from build123d import *


with BuildPart() as f1:
    # F0 (on Front) → F1 (revolve)
    with BuildSketch(Plane.XZ):
        Polygon((0, 34.925), (0, 31.75), (9.525, 31.75), (12.7, 31.75), (12.7, 34.925), (8.2938163461, 34.925), align=None)
        with BuildLine():
            Line((0, 50.8), (0, 34.925))
            Line((0, 34.925), (8.2938163461, 34.925))
            add(Edge.make_bspline(
                [(8.2938163461, 34.925), (8.8119155958, 35.9296320353), (10.3377018861, 37.6445575669), (11.8497804306, 40.251445047), (11.4775968675, 43.983221376), (10.0574266195, 46.7037851398), (7.7383380098, 48.5934290358), (5.9489654676, 49.9634460717), (3.4584093672, 50.868512047), (1.1692841349, 50.6999896772), (0, 50.8)],
                knots=[0, 0, 0, 0, 0.1331073225, 0.2566905305, 0.3928132468, 0.5191817197, 0.6423867268, 0.7502366215, 0.865279277, 1, 1, 1, 1], degree=3))
        make_face()
        with BuildLine():
            Line((0, 31.75), (0, 0))
            Line((0, 0), (19.05, 0))
            Line((19.05, 0), (19.05, 12.7))
            add(Edge.make_bspline(
                [(19.05, 12.7), (15.6508699467, 13.689246051), (10.4916904552, 17.7065910039), (7.3409641587, 20.4386906172), (6.3373062495, 26.3121345815), (10.1150269054, 30.4028265886), (9.525, 31.75)],
                knots=[0, 0, 0, 0, 0.3180499089, 0.5206308145, 0.7551272901, 1, 1, 1, 1], degree=3))
            Line((9.525, 31.75), (0, 31.75))
        make_face()
    revolve(axis=Axis((0, 0, 25.4), (0, 0, 1)))


solid = f1.part
Read the model definition and answer for the solid it produces. Units are mm, in the model's axes. A direction names the side the tool comes from. Coordinates: 2 decimals unless noted, no trailing zeros. Order: outer loops, then holes, each group sorted by start corner. A loop starts at its lowest first (then second) coordinate and runs counter-clockwise, first axis right, second up. Notation, with made-up numbers: M -5,86 L 8,86 A19 cw 8,96 Z; hole C 76.5,20 d8. An arc over 180 degrees is marked long. Put each result on its own line as item: value. Start each with the question number.
Item 1: Section A-A, the plane x = -10.5 is taken. Count the separate pieces of the cut face and the enclosed holes in it, plus the area to 3 significant figures.
Item 2: The mould has two halves that part along Z. Classify faces 3 (the face through (-2.75, -12.4, 33.36)), 4 (the face through (0, 0, 0)), 5 (the face through (-5, 9, 31.75)): +Z half, -Z half, draft (parallel to the pull), parting line (faces both ways), or undercut.
Item 3: Section B-B, the plane z = 6 is taken. Determine the outline of the cut face in (x, y), plus the area to 3 significant figures.
Item 4: Section D-D, the plane z = 33 is taken. Determine the outline of the cut face in (x, y).
Item 5: Given pin 1 Ø6 at (x, z) = (5.5, 41.5) entering from -Y; pin 2 Ø10 at (x, y) = (-12.5, -13.5) entering from +Z; pin 3 Ø6 at (x, y) = (1.5, 13.5) entering from +Z, each flat-ended and moving along its own axis, determine where each tip first touches the part or whether it passes through.
Item 6: For faces 1 (the face through (-15.12, -11.59, 6.44)), 2 (the face through (3, -8, 34.925)), determine the directions among +Z, -Z, +X, -X, +Y, -Y from which every point of the face is accessible in a straight line to the end or side of a thin tool.
Item 7: Consider probe 1 along Z at (x, y) = (-9, 5) (3 decimals); probe 2 along Z at (x, y) = (8.5, 6.5) (3 decimals); probe 3 along Y at (x, z) = (12.5, 11). Determine where each line is inside the solid, lowest interval first. Write a range as [from, to].
Computed:
1. separate pieces: 3
1. enclosed holes: 0
1. area: 600 mm2
2. face 3: draft
2. face 4: -Z half
2. face 5: undercut
3. outline: C 0,0 d38.1
3. area: 1,140 mm2
4. outline: C 0,0 d25.4
5. pin 1: stops at y = -11.35
5. pin 2: stops at z = 15.57
5. pin 3: stops at z = 45.57
6. face 1: +Z, -Z
6. face 2: none
7. probe 1: z = [0, 17.937], [31.75, 34.925], [37.768, 46.039]
7. probe 2: z = [0, 17.608], [31.75, 34.925], [38.366, 45.355]
7. probe 3: y = [-14.38, 14.38]
